CAD build for the part. Positions are in the model's coordinates, mm. Round coordinates to 2 decimals unless told otherwise and drop trailing zeros. Answer as CSV lines item,"result".
```python
from build123d import *

# Parameters (mm, degrees)
SKETCH1_W                  = 67.748
SKETCH1_H                  = 69
BOSS_EXTRUDE1_DEPTH        = 1.6
M2_5_CLEARANCE_HOLE2_D     = 3.1
M2_5_CLEARANCE_HOLE2_DEPTH = 50.8
M2_5_CLEARANCE_HOLE2_TIP   = 0.931333959
FILLET1_R                  = 2.5


with BuildPart() as part:
    # Sketch1 → Boss-Extrude1 (new body)
    with BuildSketch(Plane(origin=(0, 0, 0), x_dir=(1, 0, 0), z_dir=(0, 1, 0))):
        Rectangle(SKETCH1_W, SKETCH1_H)
    extrude(amount=BOSS_EXTRUDE1_DEPTH)

    # M2.5 Clearance Hole2
    with Locations(Plane(origin=(0, 1.6, 0), x_dir=(1, 0, 0), z_dir=(0, 1, 0))):
        with Locations((30.724, -30.453), (-30.323, 31.1), (30.727, 31.65)):
            Hole(M2_5_CLEARANCE_HOLE2_D / 2, depth=M2_5_CLEARANCE_HOLE2_DEPTH)
            with Locations((0, 0, -(M2_5_CLEARANCE_HOLE2_DEPTH + M2_5_CLEARANCE_HOLE2_TIP / 2))):  # 118° drill point
                Cone(0, M2_5_CLEARANCE_HOLE2_D / 2, M2_5_CLEARANCE_HOLE2_TIP, mode=Mode.SUBTRACT)

    # Fillet1
    fillet1_edges = [part.edges().sort_by_distance(p)[0] for p in [
        (33.874, 0.8, 34.5),
        (-33.874, 0.8, 34.5),
        (-33.874, 0.8, -34.5),
        (33.874, 0.8, -34.5),
    ]]
    fillet(fillet1_edges, radius=FILLET1_R)


solid = part.part
```
Q1. Two-plate mould, pull along Z, no slides. Class faces 1 (the flat face through (0, 0, 0)), 2 (the cylindrical face through (33.12, 0.81, 33.79)), 3 (the cylindrical face through (31.06, 0.789, 31.966)): pulls with the +Z half, pulls with the -Z half, needs draft (parallel to the pull), parting line crosses it, or undercut.
Results:
face 1,"needs draft"
face 2,"pulls with the +Z half"
face 3,"undercut"
Q2. Probe L1, parallel to X at y = 0.7, z = -31.65; L2, parallel to Z at x = 30, y = 1.55; L3, parallel to Z at x = -29, y = 1.15. List the from-to ranges inside material, lowest first. Write a range as [from, to].
Results:
L1,"[-33.87, -31.77], [-28.87, 29.18], [32.28, 33.87]"
L2,"[-34.5, -33.02], [-30.28, 29.08], [31.82, 34.5]"
L3,"[-34.5, -31.91], [-30.29, 34.5]"
Q3. Drop a flat-ended pin along its axis: pin 1 Ø5 at (x, z) = (-30.323, -31.1) entering from +Y. Give the stop position or say it passes through.
Results:
pin 1,"y = 1.6"
